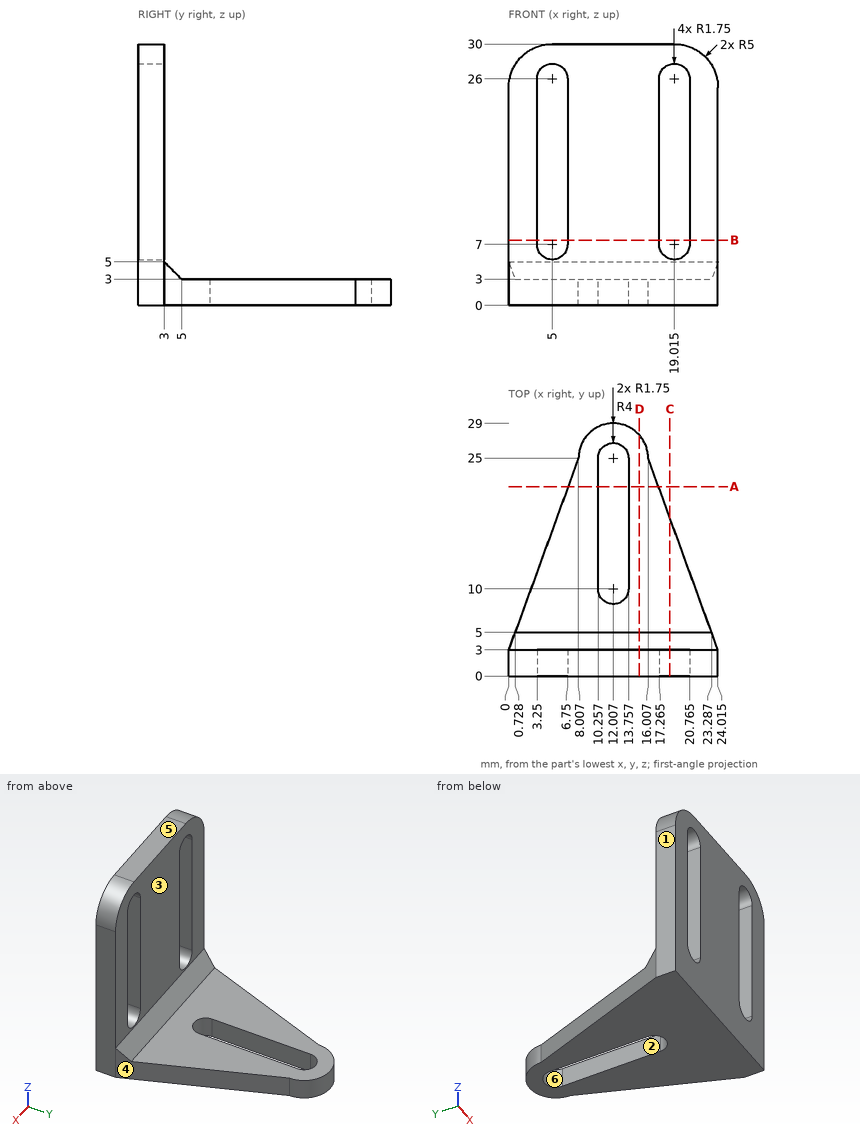
Drawing for the job (mm, zero at the part's lowest x, y, z). A direction names the side the tool comes from. Give positions to 0.01 mm unless a question says otherwise; leave off trailing zeros. Order: outer loops, then holes, each group sorted by start corner. A loop starts at its lowest first (then second) coordinate and runs counter-clockwise, first axis right, second up. Notation, with made-up numbers: M 48,54 L 53,54 A23 ccw 53,76 Z; hole C -6.5,-33.5 d11. An arc over 180 degrees is marked long. Write item = value, one per line. Start each with the question number.
(1) Which spindle directions (+Z, -Z, +X, -X, +Y, -Y) get a long thin tool onto all of the face, cutting with end or side? Do the marked faces 1, 2 and 3. Say none if no direction does.
(2) Two-plate mould, pull along Y, no slides. Class the marked faces 4, 5 and 6: released by +Y, released by -Y, zero draft, split by the parting line, or undercut.
(3) Slice it at B-B on z = 7.5. State how many separate pieces and enclosed holes the cut face has.
(4) Pin check, flat tips, straight feed: pin 1 Ø1.5 at (y, z) = (17.5, 2) entering from -X (1 decimal); pin 2 Ø11.5 at (x, y) = (14.5, 13) entering from +Z; pin 3 Ø6 at (x, z) = (21, 6.5) entering from +Y. Stop position of each tip, or through.
(5) Probe L1, parallel to Y at x = 22, z = 27.5; L2, parallel to Z at x = 12.5, y = 4.75. List the from-to ranges inside material, lowest first. Write a range as [from, to].
(6) Slice it at A-A on y = 21.75. Write the cut outline in (x, z) (1 decimal).
(7) Slice it at D-D on x = 15. Write the cut outline in (y, z), plus the area to 3 significant figures.
(8) Slice it at C-C on x = 18.5. Write the cut outline in (y, z).
Responses:
q1.face_1 = +Z, -Z, -X, +Y, -Y
q1.face_2 = +Z, -Z
q1.face_3 = +Z, +X, -X, +Y
q2.face_4 = released by +Y
q2.face_5 = zero draft
q2.face_6 = undercut
q3.separate_pieces = 3
q3.enclosed_holes = 0
q4.pin_1 = 5
q4.pin_2 = 3
q4.pin_3 = 4.5
q5.L1 = [0, 3]
q5.L2 = [0, 3.25]
q6.outline = M 6.8,0 L 10.3,0 L 10.3,3 L 6.8,3 Z; M 13.8,0 L 17.2,0 L 17.2,3 L 13.8,3 Z
q7.outline = M 0,0 L 27.65,0 L 27.65,3 L 5,3 L 3,5 L 3,30 L 0,30 Z
q7.area = 166 mm2
q8.outline = M 0,0 L 18.15,0 L 18.15,3 L 5,3 L 3,5 L 3,5.33 L 0,5.33 Z; M 0,27.67 L 3,27.67 L 3,30 L 0,30 Z
